from build123d import *

# Parameters (mm, degrees)
SKETCH1_W               = 76.2
SKETCH1_H               = 38.1
BOSS_EXTRUDE3_DEPTH     = 6.35
SKETCH3_W               = 38.1
SKETCH3_H               = 38.1
CUT_EXTRUDE1_DEPTH      = 2.54
SKETCH4_W               = 31.75
SKETCH4_H               = 38.1
BOSS_EXTRUDE4_DEPTH     = 2.54
SKETCH5_R               = 2.54
CUT_EXTRUDE5_DEPTH      = 6.35
CUT_EXTRUDE5_DEPTH_BACK = 6.35
FILLET1_R               = 5.08


with BuildPart() as part:
    # Sketch1 → Boss-Extrude3 (new body)
    with BuildSketch(Plane(origin=(0, 0, 0), x_dir=(1, 0, 0), z_dir=(0, 1, 0))):
        with Locations((38.1, 19.05)):
            Rectangle(SKETCH1_W, SKETCH1_H)
    extrude(amount=BOSS_EXTRUDE3_DEPTH)

    # Sketch3 → Cut-Extrude1 (cut)
    with BuildSketch(Plane(origin=(0, 6.35, 0), x_dir=(1, 0, 0), z_dir=(0, 1, 0))):
        with Locations((38.1, 19.05)):
            Rectangle(SKETCH3_W, SKETCH3_H)
    extrude(amount=-CUT_EXTRUDE1_DEPTH, mode=Mode.SUBTRACT)

    # Sketch4 → Boss-Extrude4 (add)
    with BuildSketch(Plane.XZ):
        with Locations((38.1, -19.05)):
            Rectangle(SKETCH4_W, SKETCH4_H)
    extrude(amount=BOSS_EXTRUDE4_DEPTH)

    # Sketch5 → Cut-Extrude5 (cut, two sides)
    with BuildSketch(Plane(origin=(0, 3.81, 0), x_dir=(1, 0, 0), z_dir=(0, 1, 0))) as cut_extrude5_sk:
        with Locations((6.35, 31.75)):
            Circle(SKETCH5_R)
        with Locations((6.35, 6.35)):
            Circle(SKETCH5_R)
        with Locations((69.85, 31.75)):
            Circle(SKETCH5_R)
        with Locations((69.85, 6.35)):
            Circle(SKETCH5_R)
    extrude(amount=CUT_EXTRUDE5_DEPTH, mode=Mode.SUBTRACT)
    extrude(cut_extrude5_sk.sketch, amount=-CUT_EXTRUDE5_DEPTH_BACK, mode=Mode.SUBTRACT)

    # Fillet1
    fillet1_edges = [part.edges().sort_by_distance(p)[0] for p in [
        (0, 3.175, -38.1),
        (0, 3.175, 0),
        (76.2, 3.175, 0),
        (76.2, 3.175, -38.1),
    ]]
    fillet(fillet1_edges, radius=FILLET1_R)


solid = part.part
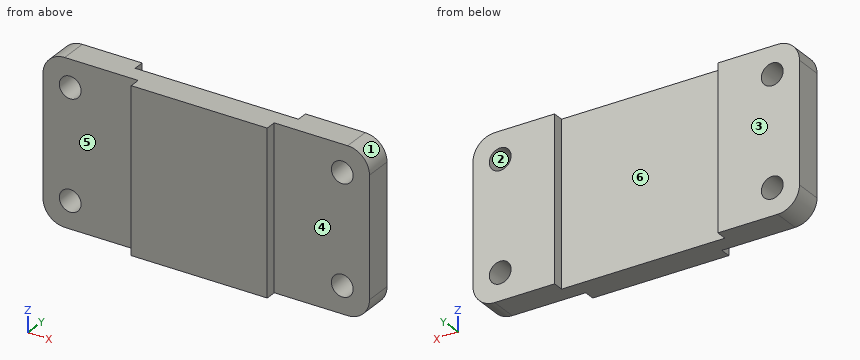
Geometry check sheet. Reference: the model listing, model coordinates, mm. Face numbers are marked on the shaded views. A direction names the side the tool comes from. Round coordinates to 2 decimals unless told otherwise and drop trailing zeros. Write each loop counter-clockwise with the first axis right and the second up, starting at its lowest first coordinate (ties: lowest second). Pieces come first, ordered by that corner, then holes. Notation, with made-up numbers: (1, 35.5) -> (45, 35.5) arc R28 cw to (45, 66.5) -> close; hole circle Ø11 at (0.25, 70.25). An arc over 180 degrees is marked (long way). One line per item, written item: value. Start each with the question number.
(1) Access from +Z, -Z, +X, -X, +Y, -Y to the whole of each face (thin tool, end or side, straight path). Record for the marked faces 4, 5 and 6.
(2) Draft check along X on the marked faces 1, 2 and 3. Enter one of: +X half, -X half, draft (parallel to the pull), parting line (faces both ways), or undercut.
(3) Cross-section at B-B, the plane y = 5.5. Record the cut outline in (x, z), and give its area (3 significant figures).
(4) Cross-section at A-A, the plane x = 69.85. Record the cut outline in (y, z).
(5) Cross-section at D-D, the plane y = 2. Record the cut outline in (x, z).
(6) Go/stop test with flat-tipped pins: pin 1 Ø2 at (y, z) = (-1.5, -23) entering from +X (3 decimals); pin 2 Ø18 at (x, z) = (8.5, -22) entering from -Y; pin 3 Ø0.8 at (y, z) = (-1.5, -21.5) entering from -X (3 decimals). Record where each tip stops, or that it passes through.
(7) Scan lines: line 1 (X direction, y = 3.5, z = -31.75); line 2 (X direction, y = 4, z = -31.75); line 3 (Z direction, x = 69.85, y = 2). Record each from-to range of solid material in increasing order. Write a range as [from, to].
(8) Cross-section at C-C, the plane z = -31.75. Record the cut outline in (x, y) (3 decimals), and give its area (3 significant figures).
Answer:
1. face 4: +Z, -Z, +X, -Y
1. face 5: +Z, -Z, -X, -Y
1. face 6: +Z, -Z, +Y
2. face 1: +X half
2. face 2: undercut
2. face 3: draft
3. outline: (0, -33.02) arc R5.08 ccw to (5.08, -38.1) -> (19.05, -38.1) -> (19.05, 0) -> (5.08, 0) arc R5.08 ccw to (0, -5.08) -> close; (57.15, -38.1) -> (71.12, -38.1) arc R5.08 ccw to (76.2, -33.02) -> (76.2, -5.08) arc R5.08 ccw to (71.12, 0) -> (57.15, 0) -> close; hole circle Ø5.08 at (6.35, -31.75); hole circle Ø5.08 at (6.35, -6.35); hole circle Ø5.08 at (69.85, -31.75); hole circle Ø5.08 at (69.85, -6.35)
3. area: 1,350 mm²
4. outline: (0, -38.1) -> (6.35, -38.1) -> (6.35, -34.29) -> (0, -34.29) -> close; (0, -29.21) -> (6.35, -29.21) -> (6.35, -8.89) -> (0, -8.89) -> close; (0, -3.81) -> (6.35, -3.81) -> (6.35, 0) -> (0, 0) -> close
5. outline: (0, -33.02) arc R5.08 ccw to (5.08, -38.1) -> (71.12, -38.1) arc R5.08 ccw to (76.2, -33.02) -> (76.2, -5.08) arc R5.08 ccw to (71.12, 0) -> (5.08, 0) arc R5.08 ccw to (0, -5.08) -> close; hole circle Ø5.08 at (6.35, -31.75); hole circle Ø5.08 at (6.35, -6.35); hole circle Ø5.08 at (69.85, -31.75); hole circle Ø5.08 at (69.85, -6.35)
6. pin 1: x = 53.975
6. pin 2: y = 0
6. pin 3: x = 22.225
7. line 1: [0, 3.81], [8.89, 67.31], [72.39, 76.2]
7. line 2: [0, 3.81], [8.89, 19.05], [57.15, 67.31], [72.39, 76.2]
7. line 3: [-38.1, -34.29], [-29.21, -8.89], [-3.81, 0]
8. outline: (0, 0) -> (3.81, 0) -> (3.81, 6.35) -> (0, 6.35) -> close; (8.89, 0) -> (22.225, 0) -> (22.225, -2.54) -> (53.975, -2.54) -> (53.975, 0) -> (67.31, 0) -> (67.31, 6.35) -> (57.15, 6.35) -> (57.15, 3.81) -> (19.05, 3.81) -> (19.05, 6.35) -> (8.89, 6.35) -> close; (72.39, 0) -> (76.2, 0) -> (76.2, 6.35) -> (72.39, 6.35) -> close
8. area: 403 mm²
